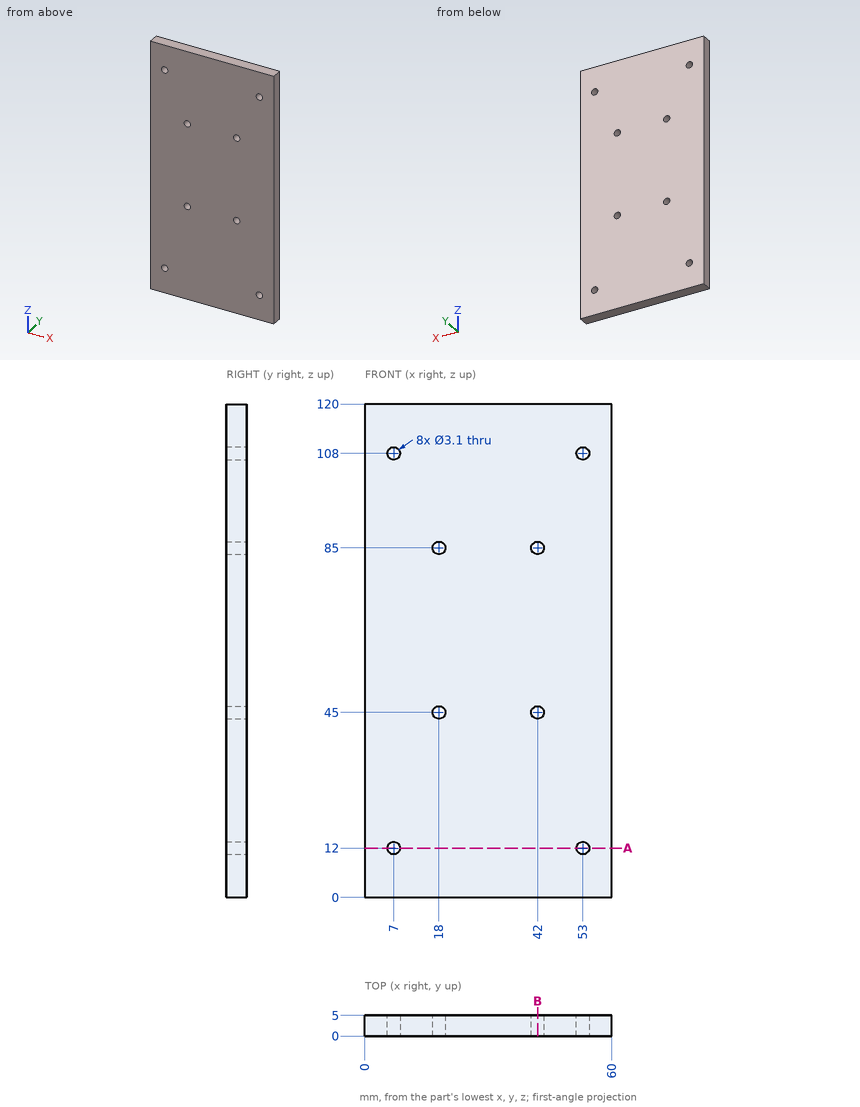
Study the drawing (mm; zero at the part's minimum x, y, z) and answer. Round coordinates to 2 decimals unless told otherwise and drop trailing zeros. Loops run counter-clockwise (first coordinate to the right, second up) from the corner with the lowest first, then second, coordinate; pieces in that order, holes last. Notation, with made-up numbers: (30.25, 53) -> (44.25, 53) arc R10 ccw to (44.25, 68) -> close; hole circle Ø2 at (6.25, 44.5). An arc over 180 degrees is marked (long way). One line per item, written item: value.
1) A flat-ended cylindrical pin translates along its axis: P1, Ø1.9, axis at x = 18, z = 45, coming from the +Y side. Find the tip coordinate at first contact, or state that the pin passes through.
Answer list:
P1: passes through
2) A cutting plane is placed at B-B (x = 42). Determine the outline of the cut face in (y, z), and give its area (3 significant figures).
Answer list:
outline: (0, 0) -> (5, 0) -> (5, 43.45) -> (0, 43.45) -> close; (0, 46.55) -> (5, 46.55) -> (5, 83.45) -> (0, 83.45) -> close; (0, 86.55) -> (5, 86.55) -> (5, 120) -> (0, 120) -> close
area: 569 mm²
3) Consider L1, parallel to Z at x = 42, y = 2.2; L2, parallel to Z at x = 7, y = 1.7; L3, parallel to X at y = 2, z = 45. Determine where each line is inside the solid, lowest interval first. Write a range as [from, to].
Answer list:
L1: z = [0, 43.45], [46.55, 83.45], [86.55, 120]
L2: z = [0, 10.45], [13.55, 106.45], [109.55, 120]
L3: x = [0, 16.45], [19.55, 40.45], [43.55, 60]
4) A cutting plane is placed at A-A (z = 12). Determine the outline of the cut face in (x, y).
Answer list:
outline: (0, 0) -> (5.45, 0) -> (5.45, 5) -> (0, 5) -> close; (8.55, 0) -> (51.45, 0) -> (51.45, 5) -> (8.55, 5) -> close; (54.55, 0) -> (60, 0) -> (60, 5) -> (54.55, 5) -> close
